CAD build for the part. Positions are in the model's coordinates, mm. Face numbers are marked on the shaded views. A direction names the side the tool comes from. Give positions to 0.01 mm unless a question says otherwise; leave off trailing zeros. Order: outer loops, then holes, each group sorted by start corner. A loop starts at its lowest first (then second) coordinate and runs counter-clockwise, first axis right, second up.
Item 1: Band-saw the part on D-D on z = -5.5. Give the cut face in (x, y).
Item 2: Which spindle directions (+Z, -Z, +X, -X, +Y, -Y) get a long thin tool onto all of the face, cutting with end or side? Do the marked faces 1, 2 and 3. Say none if no direction does.
Item 3: Band-saw the part on A-A on z = -14. Give the cut face in (x, y), plus the area to 3 significant figures.
Item 4: Band-saw the part on B-B on x = -25. Give the cut face in (y, z), plus the area to 3 significant figures.
Item 5: Flat gauge pins, fed straight in: P1, Ø10, axis at x = 47, z = -4.5, coming from the -Y side; P2, Ø16, axis at y = 71.5, z = -17, coming from the +X side; P3, Ø1.5, axis at y = -6, z = 1.5, coming from the -X side. Where does each tip first touch, or does it go through?
Item 6: Wall check: L1, parallel to Y at x = -39.5, z = -17; L2, parallel to X at y = 16.5, z = -23.5; L3, parallel to Z at x = -48.5, y = 3. Give the ranges that are in metal, low to high.
Item 7: Band-saw the part on C-C on y = -11.5. Give the cut face in (x, z).
```python
from build123d import *

# Parameters (mm, degrees)
SALIENTE_EXTRUIR1_DEPTH       = 3
CROQUIS2_R                    = 4.148409518
CROQUIS2_R_2                  = 8.791376577
CROQUIS2_R_3                  = 15.481976199
CROQUIS2_R_4                  = 8.738232185
CROQUIS2_R_5                  = 4.833412798
CORTAR_EXTRUIR1_DEPTH         = 3
CONVERTIR_S_LIDO1_START       = 3
CONVERTIR_S_LIDO1_OUTLINE_R   = 15.481976199
CONVERTIR_S_LIDO1_OUTLINE_R_2 = 8.791376577
CONVERTIR_S_LIDO1_OUTLINE_R_3 = 8.738232185
CONVERTIR_S_LIDO1_OUTLINE_R_4 = 4.148409518
CONVERTIR_S_LIDO1_OUTLINE_R_5 = 4.833412798
CONVERTIR_S_LIDO1_DEPTH       = 3
BRIDA_DE_ARISTA1_DEPTH        = 130
BRIDA_DE_ARISTA2_DEPTH        = 150


# Read off the part's stored shape, not the designer's step: Convertir-Sólido1
# Sheet-metal steps are written as plain solids
with BuildPart() as part:
    # Croquis1 → Saliente-Extruir1 (new body)
    with BuildSketch(Plane.XY):
        with BuildLine():
            Line((-53.499641927, 123.733441258), (-53.499641927, -26.266558742))
            Line((-53.499641927, -26.266558742), (76.500358073, -26.266558742))
            Line((76.500358073, -26.266558742), (76.500358073, -24.4289598))
            ThreePointArc((76.500358073, -24.4289598), (-12.000669933, 27.327433669), (-46.886740562, 123.733441258))
            Line((-46.886740562, 123.733441258), (-53.499641927, 123.733441258))
        make_face()
    extrude(amount=SALIENTE_EXTRUIR1_DEPTH)

    # Croquis2 → Cortar-Extruir1 (cut)
    with BuildSketch(Plane.XY.offset(3)):
        with Locations((28.189071336, -18.481702035)):
            Circle(CROQUIS2_R)
        with Locations((2.737394478, -9.389080565)):
            Circle(CROQUIS2_R_2)
        with Locations((-26.049076551, 10.185293851)):
            Circle(CROQUIS2_R_3)
        with Locations((-39.267642342, 40.245791579)):
            Circle(CROQUIS2_R_4)
        with Locations((-45.062734708, 65.365084268)):
            Circle(CROQUIS2_R_5)
    extrude(amount=-CORTAR_EXTRUIR1_DEPTH, mode=Mode.SUBTRACT)

    # Convertir-Sólido1 outline → Convertir-Sólido1 (add)
    with BuildSketch(Plane.XY.offset(CONVERTIR_S_LIDO1_START)):
        with BuildLine():
            Line((-53.499641927, -26.266558742), (76.500358073, -26.266558742))
            Line((76.500358073, -26.266558742), (76.500358073, -24.4289598))
            ThreePointArc((76.500358073, -24.4289598), (-12.000669933, 27.327433669), (-46.886740562, 123.733441258))
            Line((-46.886740562, 123.733441258), (-53.499641927, 123.733441258))
            Line((-53.499641927, 123.733441258), (-53.499641927, -26.266558742))
        make_face()
        with Locations((-26.049076551, 10.185293851)):
            Circle(CONVERTIR_S_LIDO1_OUTLINE_R, mode=Mode.SUBTRACT)
        with Locations((2.737394478, -9.389080565)):
            Circle(CONVERTIR_S_LIDO1_OUTLINE_R_2, mode=Mode.SUBTRACT)
        with Locations((-39.267642342, 40.245791579)):
            Circle(CONVERTIR_S_LIDO1_OUTLINE_R_3, mode=Mode.SUBTRACT)
        with Locations((28.189071336, -18.481702035)):
            Circle(CONVERTIR_S_LIDO1_OUTLINE_R_4, mode=Mode.SUBTRACT)
        with Locations((-45.062734708, 65.365084268)):
            Circle(CONVERTIR_S_LIDO1_OUTLINE_R_5, mode=Mode.SUBTRACT)
    extrude(amount=CONVERTIR_S_LIDO1_DEPTH)

    # Brida de arista1 section (across the edge) → Brida de arista1 (add)
    with BuildSketch(Plane(origin=(76.500358073, -36.266558742, 0), x_dir=(0, 1, 0), z_dir=(-1, 0, 0))):
        with BuildLine():
            Line((-6, 10), (-6, 30))
            Line((-6, 30), (0, 30))
            Line((0, 30), (0, 10))
            ThreePointArc((0, 10), (2.928932188, 2.928932188), (10, 0))
            Line((10, 0), (10, -6))
            ThreePointArc((10, -6), (-1.313708499, -1.313708499), (-6, 10))
        make_face()
    extrude(amount=BRIDA_DE_ARISTA1_DEPTH)

    # Brida de arista2 section (across the edge) → Brida de arista2 (add)
    with BuildSketch(Plane(origin=(-63.499641927, -26.266558742, 0), x_dir=(1, 0, 0), z_dir=(0, 1, 0))):
        with BuildLine():
            Line((-6, 10), (-6, 30))
            Line((-6, 30), (0, 30))
            Line((0, 30), (0, 10))
            ThreePointArc((0, 10), (2.928932188, 2.928932188), (10, 0))
            Line((10, 0), (10, -6))
            ThreePointArc((10, -6), (-1.313708499, -1.313708499), (-6, 10))
        make_face()
    extrude(amount=BRIDA_DE_ARISTA2_DEPTH)


solid = part.part
```
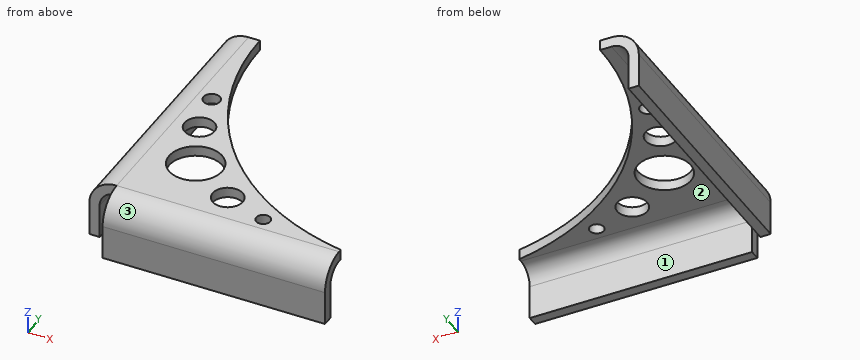
The answers:
1. outline: (-68.85, -26.27) - (-62.43, -26.27) - (-62.43, 123.73) - (-68.85, 123.73) - close; (-53.5, -41.62) - (76.5, -41.62) - (76.5, -35.2) - (-53.5, -35.2) - close
2. face 1: -Z, +X, -X, +Y
2. face 2: -Z, +X, +Y
2. face 3: +Z, +X, -X, -Y
3. outline: (-69.5, -26.27) - (-63.5, -26.27) - (-63.5, 123.73) - (-69.5, 123.73) - close; (-53.5, -42.27) - (76.5, -42.27) - (76.5, -36.27) - (-53.5, -36.27) - close
3. area: 1,680 mm2
4. outline: (-42.27, -30) - (-36.27, -30) - (-36.27, -10) arc R10 cw to (-26.27, 0) - (-5.26, 0) - (-5.26, 6) - (-26.27, 6) arc R16 ccw to (-42.27, -10) - close; (25.63, 0) - (45.53, 0) - (45.53, 6) - (25.63, 6) - close
4. area: 488 mm2
5. P1: stops at y = -42.26
5. P2: stops at x = -63.45
5. P3: stops at x = -65.35
6. L1: y = -42.27 to -36.27
6. L2: x = -69.5 to -63.5
6. L3: z = 0 to 6
7. outline: (-69.5, -30) - (-63.5, -30) - (-63.5, -10) arc R10 cw to (-53.5, 0) - (-5.8, 0) - (-5.8, 6) - (-53.5, 6) arc R16 ccw to (-69.5, -10) - close; (11.27, 0) - (37.38, 0) - (37.38, 6) - (11.27, 6) - close
